Work out the finished part from the listing and answer in its coordinate system (mm). Face numbers are marked on the shaded views. A direction names the side the tool comes from. Round coordinates to 2 decimals unless told otherwise and drop trailing zeros. Write each loop counter-clockwise with the first axis right and the second up, starting at its lowest first coordinate (ties: lowest second). Pieces come first, ordered by that corner, then holes.
1. Find section D-D (y = -43.5). Write down the section's boundary in (x, z), and give its area (3 significant figures).
2. Flat-ended cylindrical pins translate along their axes: pin 1 Ø3 at (y, z) = (-2, -0.5) entering from +X; pin 2 Ø3.5 at (x, y) = (0, 14.66) entering from -Z; pin 3 Ø3 at (y, z) = (-3.5, 0.5) entering from -X; pin 4 Ø3 at (y, z) = (-15, -1) entering from -X. Find the tip coordinate at first contact, or state that the pin passes through.
3. Find section A-A (z = -0.25). Write down the section's boundary in (x, y) (1 decimal), and give its area (3 significant figures).
4. Determine the mould class of the marked faces 3, 4, 5 and 6 for opening direction Y: pulls with the +Y half, pulls with the -Y half, needs draft (parallel to the pull), parting line crosses it, or undercut.
5. Find section C-C (x = 15.5). Write down the section's boundary in (y, z).
6. Find section B-B (y = -10). Write down the section's boundary in (x, z), and give its area (3 significant figures).
7. Straight lines are drawn through the part: probe 1 along Y at (x, z) = (3.5, 0.25); probe 2 along Y at (x, z) = (2, 1.75); probe 3 along X at (y, z) = (-8, 0.5). For each, find the intervals that lie inside material, in ascending order.
8. A tool of negligible diameter and unlimited length cuts with its end or side. For the marked faces 1 and 2, from which of +Z, -Z, +X, -X, +Y, -Y can it reach the whole face along a straight path? Write none if from no direction.
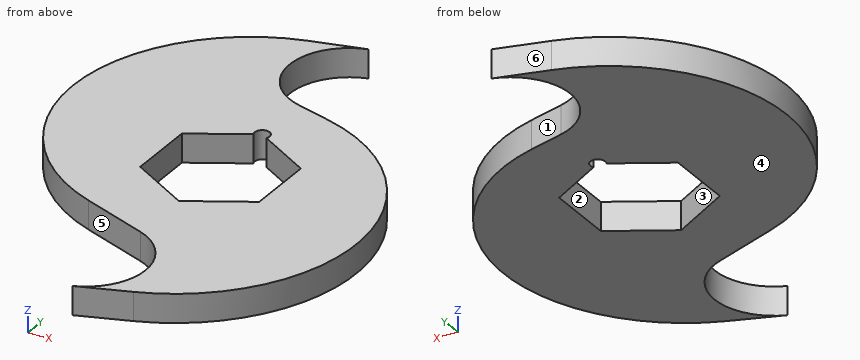
```python
from build123d import *

# Parameters (mm, degrees)
BOSS_EXTRUDE1_DEPTH = 3.048


with BuildPart() as part:
    # Sketch1 → Boss-Extrude1 (new body, symmetric)
    with BuildSketch(Plane.XY):
        with BuildLine():
            ThreePointArc((0, 27.535484012), (-9.412998127, 39.802742006), (0, 52.07))
            Line((0, 52.07), (-11.040532194, 49.111698314))
            ThreePointArc((-11.040532194, 49.111698314), (-39.066320922, 14.192289272), (-14.190605813, -23.03684931))
            Line((-14.190605813, -23.03684931), (0, -28.201807432))
            ThreePointArc((0, -28.201807432), (8.35634418, -40.135903716), (0, -52.07))
            Line((0, -52.07), (10.740686656, -48.160709762))
            ThreePointArc((10.740686656, -48.160709762), (36.144496882, -10.141220984), (7.52373904, 25.519504212))
            Line((7.52373904, 25.519504212), (0, 27.535484012))
        make_face()
        with BuildLine():
            Line((-12.7, 7.332348419), (-1.374815329, 13.870946837))
            ThreePointArc((-1.374815329, 13.870946837), (-0.410875234, 16.198104087), (1.5875, 14.664696837))
            ThreePointArc((1.5875, 14.664696837), (1.533407249, 14.253821603), (1.374815329, 13.870946837))
            Line((1.374815329, 13.870946837), (12.7, 7.332348419))
            Line((12.7, 7.332348419), (12.7, -7.332348419))
            Line((12.7, -7.332348419), (0, -14.664696837))
            Line((0, -14.664696837), (-12.7, -7.332348419))
            Line((-12.7, -7.332348419), (-12.7, 7.332348419))
        make_face(mode=Mode.SUBTRACT)
    extrude(amount=BOSS_EXTRUDE1_DEPTH, both=True)


solid = part.part
```
Worked answers:
1. outline: (7.9, -3.05) - (19.69, -3.05) - (19.69, 3.05) - (7.9, 3.05) - close
1. area: 71.9 mm2
2. pin 1: stops at x = 35.27
2. pin 2: stops at z = -3.05
2. pin 3: stops at x = -36.2
2. pin 4: stops at x = -28.72
3. outline: (-14.2, -23) - (0, -28.2) arc R12.7 cw to (0, -52.1) - (10.7, -48.2) arc R38.7 ccw to (7.5, 25.5) - (0, 27.5) arc R12.7 cw to (0, 52.1) - (-11, 49.1) arc R37.9 ccw to start; hole (-12.7, -7.3) - (0, -14.7) - (12.7, -7.3) - (12.7, 7.3) - (1.4, 13.9) arc R1.6 ccw (long way) to (-1.4, 13.9) - (-12.7, 7.3) - close
3. area: 3,650 mm2
4. face 3: undercut
4. face 4: needs draft
4. face 5: pulls with the -Y half
4. face 6: pulls with the +Y half
5. outline: (-46.06, -3.05) - (22.4, -3.05) - (22.4, 3.05) - (-46.06, 3.05) - close
6. outline: (-31.66, -3.05) - (-8.08, -3.05) - (-8.08, 3.05) - (-31.66, 3.05) - close; (8.08, -3.05) - (36.14, -3.05) - (36.14, 3.05) - (8.08, 3.05) - close
6. area: 315 mm2
7. probe 1: y = -50.8 to -50.12, -30.15 to -12.64, 12.64 to 26.6
7. probe 2: y = -51.34 to -51.14, -29.13 to -13.51, 13.51 to 27
7. probe 3: x = -33.05 to -11.54, 11.54 to 35.99
8. face 1: +Z, -Z, +X, +Y
8. face 2: +Z, -Z
